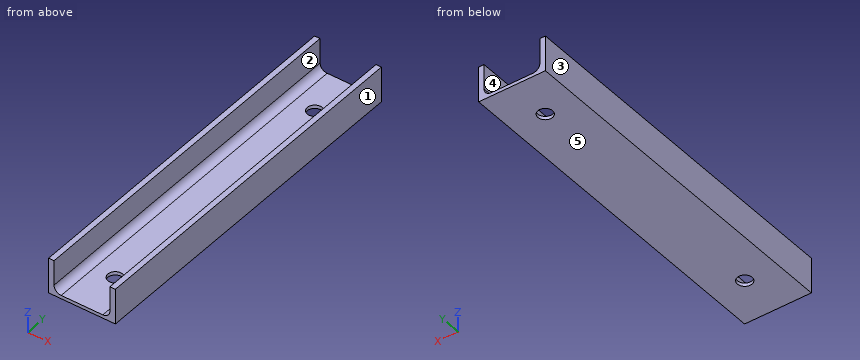
from build123d import *

# Parameters (mm, degrees)
F1_DEPTH = 400
F3_D     = 16.5


with BuildPart() as f1:
    # F0 (on Front) → F1 (new body)
    with BuildSketch(Plane.XZ):
        with BuildLine():
            Line((-37.5, 0), (0, 0))
            Line((0, 0), (37.5, 0))
            Line((37.5, 0), (37.5, 40))
            Line((37.5, 40), (31.4, 40))
            Line((31.4, 40), (31.4, 11.8))
            ThreePointArc((31.4, 11.8), (29.0568542495, 6.1431457505), (23.4, 3.8))
            Line((23.4, 3.8), (0, 3.8))
            Line((0, 3.8), (-23.4, 3.8))
            ThreePointArc((-23.4, 3.8), (-29.0568542495, 6.1431457505), (-31.4, 11.8))
            Line((-31.4, 11.8), (-31.4, 40))
            Line((-31.4, 40), (-37.5, 40))
            Line((-37.5, 40), (-37.5, 0))
        make_face()
    extrude(amount=F1_DEPTH)

    # F3 (through all)
    with Locations(Plane(origin=(0, 0, 0), x_dir=(1, 0, 0), z_dir=(0, 0, -1))):
        with Locations((0, 50), (0, 350)):
            Hole(F3_D / 2)


solid = f1.part
Geometry: final body of the model. Coordinates: model frame, mm. Face numbers are marked on the shaded views. A direction names the side the tool comes from. Give positions to 0.01 mm unless a question says otherwise; leave off trailing zeros. Write each loop counter-clockwise with the first axis right and the second up, starting at its lowest first coordinate (ties: lowest second). Pieces come first, ordered by that corner, then holes.
(1) Cut plane C-C, the plane x = 0. Return loops of the section in (y, z).
(2) Cut plane A-A, the plane y = -50. Return loops of the section in (x, z), then the cut area to 3 significant figures.
(3) Cut plane D-D, the plane y = -141. Return loops of the section in (x, z), then the cut area to 3 significant figures.
(4) First-contact query: P1, Ø10, axis at x = -13.5, z = 7.5, coming from the +Y side; P2, Ø10, axis at x = -24, z = 27.5, coming from the +Y side; P3, Ø1, axis at x = -18, y = -170, coming from the +Z side. Flat tips, straight axial feed; report the tip coordinate or a pass-through.
(5) Ray query, line 1 (Y direction, x = 0, z = 1.9); line 2 (X direction, y = -77.5, z = 31.5); line 3 (X direction, y = -50, z = 0.9). Return the intervals inside material, ascending.
(6) Cut plane B-B, the plane z = 20. Return loops of the section in (x, y), then the cut area to 3 significant figures.
(7) Access query for the marked faces 1 and 2. Directions: +Z, -Z, +X, -X, +Y, -Y. A direction counts if a zero-diameter tool reaches every point of the face in a straight line with its end or side. Return the directions, or none.
(8) Mould query, pull axis X, two halves, no side actions, for the marked faces 3, 4 and 5. Classes: released by +X, released by -X, zero draft, split by the parting line, or undercut.
Values follow:
1. outline: (-400, 0) - (-358.25, 0) - (-358.25, 3.8) - (-400, 3.8) - close; (-341.75, 0) - (-58.25, 0) - (-58.25, 3.8) - (-341.75, 3.8) - close; (-41.75, 0) - (0, 0) - (0, 3.8) - (-41.75, 3.8) - close
2. outline: (-37.5, 0) - (-8.25, 0) - (-8.25, 3.8) - (-23.4, 3.8) arc R8 cw to (-31.4, 11.8) - (-31.4, 40) - (-37.5, 40) - close; (8.25, 0) - (37.5, 0) - (37.5, 40) - (31.4, 40) - (31.4, 11.8) arc R8 cw to (23.4, 3.8) - (8.25, 3.8) - close
2. area: 691 mm2
3. outline: (-37.5, 0) - (37.5, 0) - (37.5, 40) - (31.4, 40) - (31.4, 11.8) arc R8 cw to (23.4, 3.8) - (-23.4, 3.8) arc R8 cw to (-31.4, 11.8) - (-31.4, 40) - (-37.5, 40) - close
3. area: 754 mm2
4. P1: stops at y = 0
4. P2: passes through
4. P3: stops at z = 3.8
5. line 1: y = -400 to -358.25, -341.75 to -58.25, -41.75 to 0
5. line 2: x = -37.5 to -31.4, 31.4 to 37.5
5. line 3: x = -37.5 to -8.25, 8.25 to 37.5
6. outline: (-37.5, -400) - (-31.4, -400) - (-31.4, 0) - (-37.5, 0) - close; (31.4, -400) - (37.5, -400) - (37.5, 0) - (31.4, 0) - close
6. area: 4,880 mm2
7. face 1: +Z, -Z, +X, +Y, -Y
7. face 2: +Z, +Y, -Y
8. face 3: released by -X
8. face 4: undercut
8. face 5: zero draft
